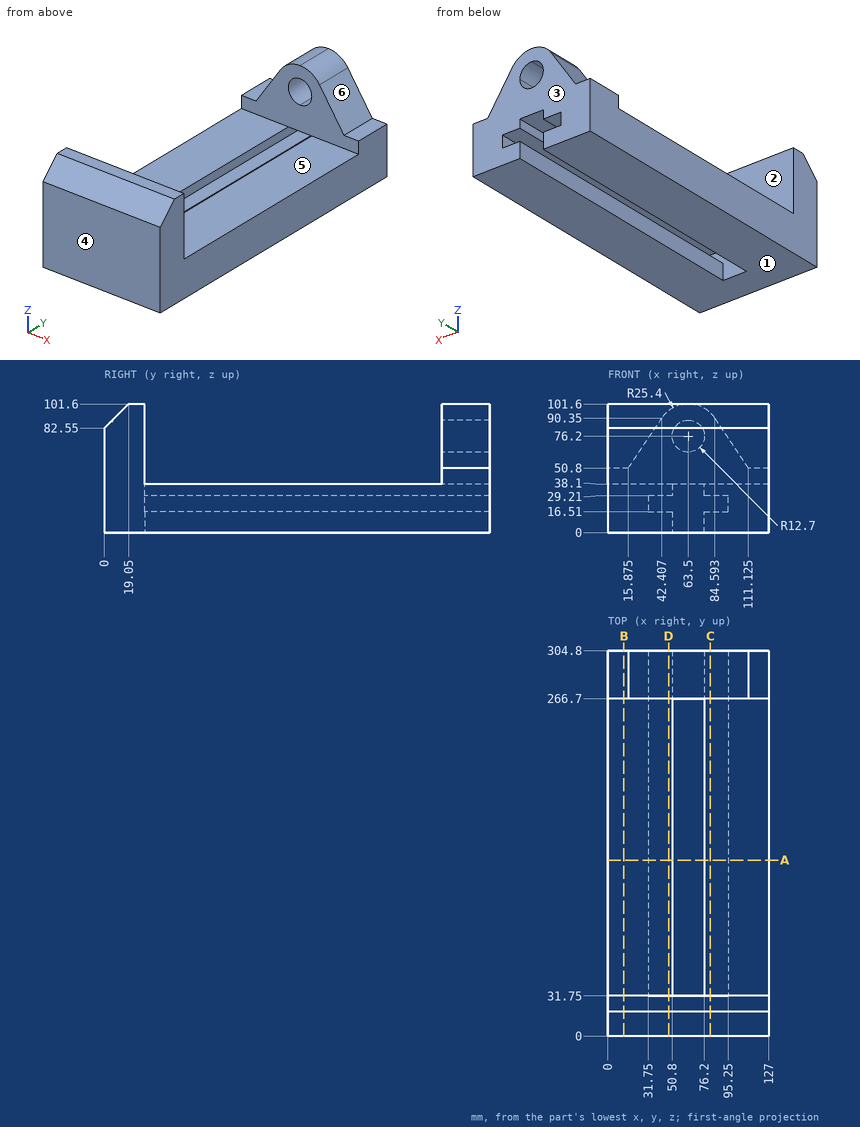
Study the drawing (mm; zero at the part's minimum x, y, z) and answer. A direction names the side the tool comes from. Give positions to 0.01 mm unless a question says otherwise; leave off trailing zeros. Loops run counter-clockwise (first coordinate to the right, second up) from the corner with the lowest first, then second, coordinate; pieces in that order, holes last. Notation, with made-up numbers: (21, 48.25) - (30, 48.25) arc R9 cw to (30, 63.25) - close; hole circle Ø1 at (75, -2). An arc over 180 degrees is marked (long way). Answer as CSV lines item,"result". Start each with the question number.
1) Each of these flat-tipped pins is pushed along its axis until it touches: pin 1 Ø8 at (x, y) = (120, 294) entering from +Z; pin 2 Ø17.5 at (x, y) = (7.5, 287) entering from +Z; pin 3 Ø6 at (x, y) = (87, 50) entering from +Z. Where does it stop, or does it pass through?
2) Straight lines are drawn through the part: L1, parallel to X at y = 73, z = 15; L2, parallel to Z at x = 89, y = 156; L3, parallel to Y at x = 97, z = 59. For each, find the intervals that lie inside material, in ascending order. Write a range as from..to.
3) Find section B-B (x = 12.5). Write down the section's boundary in (y, z), then the cut area to 3 significant figures.
4) Determine the mould class of the marked faces 1, 2 and 3 for opening direction Y: released by +Y, released by -Y, zero draft, split by the parting line, or undercut.
5) Find section C-C (x = 81). Write down the section's boundary in (y, z), then the cut area to 3 significant figures.
6) Which of the six approach directions +Z, -Z, +X, -X, +Y, -Y give full straight-line access (tool end or side, diameter ignored) to the marked faces 4, 5 and 6?
7) Find section D-D (x = 48). Write down the section's boundary in (y, z).
8) Find section A-A (y = 139). Write down the section's boundary in (x, z), then the cut area to 3 significant figures.
Findings below:
1,pin 1,"z = 50.8"
1,pin 2,"z = 51.36"
1,pin 3,"z = 38.1"
2,L1,"0..50.8, 76.2..127"
2,L2,"0..16.51, 29.21..38.1"
2,L3,"0..31.75, 266.7..304.8"
3,outline,"(0, 0) - (304.8, 0) - (304.8, 50.8) - (266.7, 50.8) - (266.7, 38.1) - (31.75, 38.1) - (31.75, 101.6) - (19.05, 101.6) - (0, 82.55) - close"
3,area,"13,900 mm^2"
4,face 1,"zero draft"
4,face 2,"undercut"
4,face 3,"released by +Y"
5,outline,"(0, 0) - (304.8, 0) - (304.8, 16.51) - (31.75, 16.51) - (31.75, 29.21) - (304.8, 29.21) - (304.8, 94.61) - (266.7, 94.61) - (266.7, 38.1) - (31.75, 38.1) - (31.75, 101.6) - (19.05, 101.6) - (0, 82.55) - close"
5,area,"12,100 mm^2"
6,face 4,"+Z, -Z, +X, -X, -Y"
6,face 5,"+Z, +X, -X"
6,face 6,"+Z, +X, +Y"
7,outline,"(0, 0) - (304.8, 0) - (304.8, 16.51) - (31.75, 16.51) - (31.75, 29.21) - (304.8, 29.21) - (304.8, 96.32) - (266.7, 96.32) - (266.7, 38.1) - (31.75, 38.1) - (31.75, 101.6) - (19.05, 101.6) - (0, 82.55) - close"
8,outline,"(0, 0) - (50.8, 0) - (50.8, 16.51) - (31.75, 16.51) - (31.75, 29.21) - (50.8, 29.21) - (50.8, 38.1) - (0, 38.1) - close; (76.2, 0) - (127, 0) - (127, 38.1) - (76.2, 38.1) - (76.2, 29.21) - (95.25, 29.21) - (95.25, 16.51) - (76.2, 16.51) - close"
8,area,"3,390 mm^2"
